```python
from build123d import *

# Parameters (mm, degrees)
SKETCH1_R           = 50
BOSS_EXTRUDE1_DEPTH = 3.175
SKETCH3_R           = 7.5
CUT_EXTRUDE1_DEPTH  = 71.78192301
FILLET3_R           = 0.127
SKETCH4_R           = 5
BOSS_EXTRUDE2_DEPTH = 10


with BuildPart() as part:
    # Sketch1 → Boss-Extrude1 (new body)
    with BuildSketch(Plane(origin=(0, 0, 0), x_dir=(1, 0, 0), z_dir=(0, 1, 0))):
        with Locations(Location((0, 0, 0), (0, 0, 270))):
            Circle(SKETCH1_R)
    extrude(amount=BOSS_EXTRUDE1_DEPTH)

    # Sketch3 → Cut-Extrude1 (cut, through all)
    with BuildSketch(Plane(origin=(0, 3.175, 0), x_dir=(1, 0, 0), z_dir=(0, 1, 0))):
        with Locations(Location((0, 0, 0), (0, 0, 270))):
            Circle(SKETCH3_R)
    extrude(amount=-CUT_EXTRUDE1_DEPTH, mode=Mode.SUBTRACT)

    # Fillet3
    fillet3_edges = [part.edges().sort_by_distance(p)[0] for p in [
        (0, 0, -7.5),
        (0, 3.175, -7.5),
    ]]
    fillet(fillet3_edges, radius=FILLET3_R)

    # Sketch4 → Boss-Extrude2 (add)
    with BuildSketch(Plane(origin=(0, 3.175, 0), x_dir=(1, 0, 0), z_dir=(0, 1, 0))):
        with Locations(Location((0, 42, 0), (0, 0, 270))):
            Circle(SKETCH4_R)
    extrude(amount=BOSS_EXTRUDE2_DEPTH)


solid = part.part
```
Here's how the part is built. I have some questions about the finished solid (model axes, mm). A direction names the side the tool comes from. Coordinates: 2 decimals unless noted, no trailing zeros. Order: outer loops, then holes, each group sorted by start corner. A loop starts at its lowest first (then second) coordinate and runs counter-clockwise, first axis right, second up. Notation, with made-up numbers: M -37,82.5 L -18,82.5 A19 cw -18,113.5 Z; hole C 48.5,63 d1. An arc over 180 degrees is marked long. Answer as a JSON object with one key per item and string values. Group by question number.
(1) Suppose I cut it at C-C, the plane y = 5.75. Please give me the cut outline in (x, z).
(2) Suppose I cut it at A-A, the plane z = 0. Please give me the cut outline in (x, y) (3 decimals), then the cut area to 3 significant figures.
(3) If we mould it in two halves opening along Z, with no side actions, what happens to faces 3 (the face through (0.33, 1.608, -7.493)), 4 (the face through (0, 13.175, -42)), 5 (the face through (15.02, 1.57, 47.69))? For each: released by +Z, released by -Z, zero draft, split by the parting line, or undercut.
(4) For pin 1 (2 mm diameter, centred on x = 5.5, z = 24.5, fed in from -Y); pin 2 (4 mm diameter, centred on x = 28, z = -0.5, fed in from +Y) (3 decimals); pin 3 (2 mm diameter, centred on x = 18, y = 3.5, fed in from -Z), each with a flat end and sliding along its axis, tell me the tip position at first contact or that it passes through.
(5) Suppose I cut it at B-B, the plane x = 0. Please give me the cut outline in (y, z) (3 decimals).
(6) I need wall thicknesses on probe 1 along X at (y, z) = (2.5, 0); probe 2 along Y at (x, z) = (-20, 23) (3 decimals); probe 3 along X at (y, z) = (2, 5). Which ranges of each line are inside material? Lowest first, please.
(7) Which directions (+Z, -Z, +X, -X, +Y, -Y) give clear straight access to the entire face, cutting with the end or side of a thin tool? Please do faces 1 (the face through (-10, 0, -1)), 2 (the face through (0, 8, -47)).
(8) Suppose I cut it at D-D, the plane z = -42. Please give me the cut outline in (x, y) (3 decimals).
Values found:
{
 "1": {"outline": "C 0,-42 d10"},
 "2": {"outline": "M -50,0 L -7.627,0 A0.127 ccw -7.5,0.127 L -7.5,3.048 A0.127 ccw -7.627,3.175 L -50,3.175 Z; M 7.5,0.127 A0.127 ccw 7.627,0 L 50,0 L 50,3.175 L 7.627,3.175 A0.127 ccw 7.5,3.048 Z", "area": "270 mm^2"},
 "3": {"face 3": "undercut", "face 4": "zero draft", "face 5": "split by the parting line"},
 "4": {"pin 1": "stops at y = 0", "pin 2": "stops at y = 3.175", "pin 3": "stops at z = -47"},
 "5": {"outline": "M 0,-50 L 3.175,-50 L 3.175,-47 L 13.175,-47 L 13.175,-37 L 3.175,-37 L 3.175,-7.627 A0.127 ccw 3.048,-7.5 L 0.127,-7.5 A0.127 ccw 0,-7.627 Z; M 0,7.627 A0.127 ccw 0.127,7.5 L 3.048,7.5 A0.127 ccw 3.175,7.627 L 3.175,50 L 0,50 Z"},
 "6": {"probe 1": "x = -50 to -7.5, 7.5 to 50", "probe 2": "y = 0 to 3.175", "probe 3": "x = -49.75 to -5.59, 5.59 to 49.75"},
 "7": {"face 1": "+Z, -Z, +X, -X, -Y", "face 2": "+Y"},
 "8": {"outline": "M -27.129,0 L 27.129,0 L 27.129,3.175 L 5,3.175 L 5,13.175 L -5,13.175 L -5,3.175 L -27.129,3.175 Z"}
}
